```python
from build123d import *

# Parameters (mm, degrees)
SKETCH1_W             = 17
SKETCH1_H             = 17
BOSS_EXTRUDE1_DEPTH   = 8
SKETCH2_W             = 5
SKETCH2_H             = 4
BOSS_EXTRUDE2_DEPTH   = 3.5
SKETCH3_W             = 5
SKETCH3_H             = 4
BOSS_EXTRUDE3_DEPTH   = 3.5
M2X0_4_TAPPED_HOLE1_D = 1.6
FILLET1_R             = 2
SKETCH8_R             = 7.5
BOSS_EXTRUDE4_DEPTH   = 7
SKETCH9_R             = 6
CUT_EXTRUDE1_DEPTH    = 16
FILLET2_R             = 0.2


with BuildPart() as part:
    # Sketch1 → Boss-Extrude1 (new body)
    with BuildSketch(Plane(origin=(0, 0, 0), x_dir=(1, 0, 0), z_dir=(0, 1, 0))):
        Rectangle(SKETCH1_W, SKETCH1_H)
    extrude(amount=BOSS_EXTRUDE1_DEPTH)

    # Sketch2 → Boss-Extrude2 (add)
    with BuildSketch(Plane.XY.offset(8.5)):
        with Locations((0, 2)):
            Rectangle(SKETCH2_W, SKETCH2_H)
    extrude(amount=BOSS_EXTRUDE2_DEPTH)

    # Sketch3 → Boss-Extrude3 (add)
    with BuildSketch(Plane(origin=(0, 0, -8.5), x_dir=(-1, 0, 0), z_dir=(0, 0, -1))):
        with Locations((0, 2)):
            Rectangle(SKETCH3_W, SKETCH3_H)
    extrude(amount=BOSS_EXTRUDE3_DEPTH)

    # M2x0.4 Tapped Hole1 (through all)
    with Locations(Plane(origin=(0, 4, 0), x_dir=(1, 0, 0), z_dir=(0, 1, 0))):
        with Locations((0, -10), (0, 10)):
            Hole(M2X0_4_TAPPED_HOLE1_D / 2)

    # Fillet1
    fillet1_edges = [part.edges().sort_by_distance(p)[0] for p in [
        (-2.5, 2, 12),
        (2.5, 2, 12),
        (-2.5, 2, -12),
        (2.5, 2, -12),
    ]]
    fillet(fillet1_edges, radius=FILLET1_R)

    # Sketch8 → Boss-Extrude4 (add)
    with BuildSketch(Plane(origin=(0, 8, 0), x_dir=(1, 0, 0), z_dir=(0, 1, 0))):
        Circle(SKETCH8_R)
    extrude(amount=BOSS_EXTRUDE4_DEPTH)

    # Sketch9 → Cut-Extrude1 (cut, through all)
    with BuildSketch(Plane(origin=(0, 15, 0), x_dir=(1, 0, 0), z_dir=(0, 1, 0))):
        Circle(SKETCH9_R)
    extrude(amount=-CUT_EXTRUDE1_DEPTH, mode=Mode.SUBTRACT)

    # Fillet2
    fillet2_edges = [part.edges().sort_by_distance(p)[0] for p in [
        (-7.5, 15, 0),
        (8.5, 4, 8.5),
        (8.5, 4, -8.5),
        (-8.5, 4, 8.5),
        (-8.5, 4, -8.5),
        (2.5, 4, 9.25),
        (1.914213562, 4, 11.414213562),
        (-1.914213562, 4, 11.414213562),
        (-2.5, 4, 9.25),
        (0, 8, 8.5),
        (8.5, 8, 0),
        (-8.5, 8, 0),
        (0, 8, -8.5),
        (2.5, 4, -9.25),
        (1.914213562, 4, -11.414213562),
        (-1.914213562, 4, -11.414213562),
        (-2.5, 4, -9.25),
        (0, 4, 12),
        (0, 4, -12),
    ]]
    fillet(fillet2_edges, radius=FILLET2_R)


solid = part.part
```
Here's how the part is built. I have some questions about the finished solid (model axes, mm). A direction names the side the tool comes from. Coordinates: 2 decimals unless noted, no trailing zeros. Write each loop counter-clockwise with the first axis right and the second up, starting at its lowest first coordinate (ties: lowest second). Pieces come first, ordered by that corner, then holes. Notation, with made-up numbers: (-38, 89.25) - (-33, 89.25) arc R20 cw to (-33, 109.25) - close; hole circle Ø10 at (52.25, 41.25). An arc over 180 degrees is marked (long way). One line per item, written item: value.
1) I need wall thicknesses on line 1 along Z through (x, y) = (0, 1.75); line 2 along X through (y, z) = (3.25, 0); line 3 along X through (y, z) = (8.75, 0). Which ranges of each line are inside material? Lowest first, please.
Model answer:
line 1: z = -12 to -10.8, -9.2 to -6, 6 to 9.2, 10.8 to 12
line 2: x = -8.5 to -6, 6 to 8.5
line 3: x = -7.5 to -6, 6 to 7.5
2) I'm going to push flat-ended pins straight in: P1, Ø2.5, axis at x = -1, z = 9.5, coming from the +Y side; P2, Ø2.5, axis at x = -3.5, y = 3, coming from the +Z side; P3, Ø0.8, axis at y = 1, z = -9.5, coming from the -X side. Where does each tip first touch, or does it pass through?
Model answer:
P1: stops at y = 8
P2: stops at z = 10.97
P3: stops at x = -2.5
3) On a 3-axis mill with a long thin cutter (end or side, diameter ignored), from which of +Z, -Z, +X, -X, +Y, -Y can I reach the whole of each face in a straight line? I mean faces 1 (the flat face through (-2.5, 2, -9)), 2 (the flat face through (2.5, 2, -9)), 3 (the flat face through (2.5, 2, 9)), 4 (the flat face through (-2.5, 2, 9)), 5 (the flat face through (0, 5, -8.5)). Say none if no direction works.
Model answer:
face 1: -Z, -X, +Y, -Y
face 2: -Z, +X, +Y, -Y
face 3: +Z, +X, +Y, -Y
face 4: +Z, -X, +Y, -Y
face 5: -Z, +Y
4) Suppose I cut it at B-B on z = 0. Write out the boundary of the cut face in (x, y), and give its area (3 significant figures).
Model answer:
outline: (-8.5, 0) - (-6, 0) - (-6, 15) - (-7.3, 15) arc R0.2 ccw to (-7.5, 14.8) - (-7.5, 8) - (-8.3, 8) arc R0.2 ccw to (-8.5, 7.8) - close; (6, 0) - (8.5, 0) - (8.5, 7.8) arc R0.2 ccw to (8.3, 8) - (7.5, 8) - (7.5, 14.8) arc R0.2 ccw to (7.3, 15) - (6, 15) - close
area: 61.0 mm²
5) Suppose I cut it at A-A on x = 0. State how many separate pieces and enclosed holes the cut face has, and give its area (3 significant figures).
Model answer:
separate pieces: 4
enclosed holes: 0
area: 76.1 mm²
6) Suppose I cut it at C-C on y = 9.75. Write out the boundary of the cut face in (x, z), and give its area (3 significant figures).
Model answer:
outline: circle Ø15 at (0, 0); hole circle Ø12 at (0, 0)
area: 63.6 mm²
7) We'd pull the mould along X, two halves only. Please class faces 6 (the cylindrical face through (0.104, 1.972, 9.207)), 7 (the flat face through (-6, 0, -3)), 8 (the cylindrical face through (-1.93, 1.93, 11.4)), 9 (the cylindrical face through (-7.493, 11.352, -0.33)): pulls with the +X half, pulls with the -X half, needs draft (parallel to the pull), parting line crosses it, or undercut.
Model answer:
face 6: undercut
face 7: needs draft
face 8: pulls with the -X half
face 9: parting line crosses it
